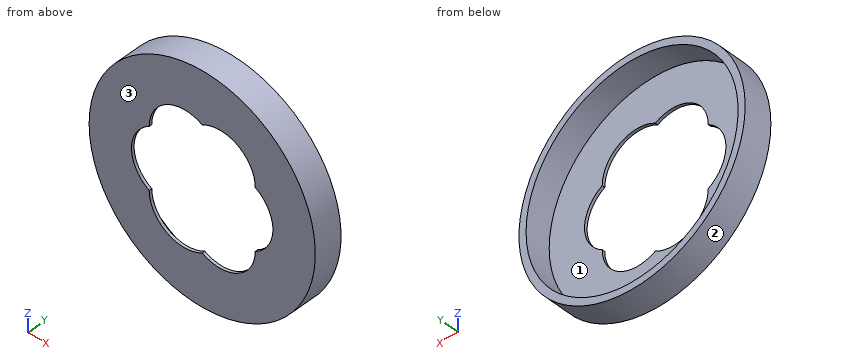
Autodesk Inventor part; units mm, degrees
ref_plane "YZ Plane" through (0, 0, 0) normal (1, 0, 0) x (0, 1, 0)
ref_plane "XZ Plane" through (0, 0, 0) normal (0, 1, 0) x (-1, 0, 0)
ref_plane "XY Plane" through (0, 0, 0) normal (0, 0, 1) x (1, 0, 0)
sketch "Sketch1" plane through (0, 0, 0) normal (0, 1, 0) x (-1, 0, 0)
  circle A0 centre (0, 0) radius 20.32
  dimension "d0" = 40.64
extrude "Extrusion1" add sketch "Sketch1" along normal blind 5.08
sketch "Sketch2" plane through (0, 5.08, 0) normal (0, 1, 0) x (1, 0, 0)
  circle A0 centre (0, 0) radius 19.05
  dimension "d3" = 38.1
extrude "Extrusion2" cut sketch "Sketch2" against normal blind 4.572
sketch "Sketch3" plane through (0, 0.508, 0) normal (0, 1, 0) x (1, 0, 0)
  line L0 (0, 0) -> (-6.35, 0)
  circle A0 centre (-6.35, 0) radius 6.35
  dimension "d6" = 6.35
extrude "Extrusion3" cut sketch "Sketch3" against normal blind 4.572
pattern_circular "Circular Pattern1" count 6 over 360 about axis through (0, 0.508, 0) along (0, 1, 0) of "Extrusion3"
sketch "Sketch4" plane through (0, 0.508, 0) normal (0, 1, 0) x (1, 0, 0)
  line L0 (0, 0) -> (-6.35, 0)
  dimension "d14" = 6.35
properties part number "Motor Mount Test"
Geometry check sheet. Reference: the model listing, model coordinates, mm. Face numbers are marked on the shaded views. Give positions to 0.01 mm unless a question says otherwise; leave off trailing zeros. Order: outer loops, then holes, each group sorted by start corner. A loop starts at its lowest first (then second) coordinate and runs counter-clockwise, first axis right, second up. Notation, with made-up numbers: (19, -26) - (35, -26) arc R13 cw to (35, -20) - close; hole circle Ø9 at (34.5, 8.25). An arc over 180 degrees is marked (long way). Answer in a Markdown table with one row per item. Add a question column.
Q1. Mould release check, pull along Z, two halves, no side actions. Record for the marked faces 1, 2 and 3: pulls with the +Z half, pulls with the -Z half, needs draft (parallel to the pull), parting line crosses it, or undercut.
Q2. Cross-section at A-A, the plane z = 0. Enter the section's corners in (x, y).
Q3. Gauge pin test, flat ends, axial feed: pin 1 (2 mm diameter, centred on y = 1, z = 12.5, fed in from -X); pin 2 (1.5 mm diameter, centred on y = 4, z = 6, fed in from +X); pin 3 (1.5 mm diameter, centred on y = 1, z = 10.5, fed in from +X). Record the tip position at first contact, or that the pin passes through.
Q4. Cross-section at C-C, the plane y = 1.35. Enter the section's corners in (x, z).
Q5. Material ranges on probe 1 along X at (y, z) = (3.9, -16.5); probe 2 along Z at (x, y) = (0, 1.7); probe 3 along Y at (x, z) = (-14, 9.5), recorded low to high. Write a range as from..to.
Q6. Cross-section at D-D, the plane x = 18. Enter the section's corners in (y, z), then the cut area to 3 significant figures.
Q7. Cross-section at B-B, the plane x = -4.5. Enter the section's corners in (y, z), then the cut area to 3 significant figures.
Check values:
| question | item | result |
|---|---|---|
| 1 | face 1 | undercut |
| 1 | face 2 | parting line crosses it |
| 1 | face 3 | needs draft |
| 2 | outline | (-20.32, 0) - (-12.7, 0) - (-12.7, 0.51) - (-19.05, 0.51) - (-19.05, 5.08) - (-20.32, 5.08) - close; (12.7, 0) - (20.32, 0) - (20.32, 5.08) - (19.05, 5.08) - (19.05, 0.51) - (12.7, 0.51) - close |
| 3 | pin 1 | stops at x = -16.75 |
| 3 | pin 2 | stops at x = 19.63 |
| 3 | pin 3 | stops at x = 17.83 |
| 4 | outline | circle Ø40.64 at (0, 0); hole circle Ø38.1 at (0, 0) |
| 5 | probe 1 | x = -11.86..-9.52, 9.52..11.86 |
| 5 | probe 2 | z = -20.32..-19.05, 19.05..20.32 |
| 5 | probe 3 | y = 0..0.51 |
| 6 | outline | (0, -9.43) - (5.08, -9.43) - (5.08, -6.24) - (0.51, -6.24) - (0.51, 6.24) - (5.08, 6.24) - (5.08, 9.43) - (0, 9.43) - close |
| 6 | area | 38.8 mm^2 |
| 7 | outline | (0, -19.82) - (5.08, -19.82) - (5.08, -18.51) - (0.51, -18.51) - (0.51, -11.71) - (0, -11.71) - close; (0, 11.71) - (0.51, 11.71) - (0.51, 18.51) - (5.08, 18.51) - (5.08, 19.82) - (0, 19.82) - close |
| 7 | area | 20.2 mm^2 |
